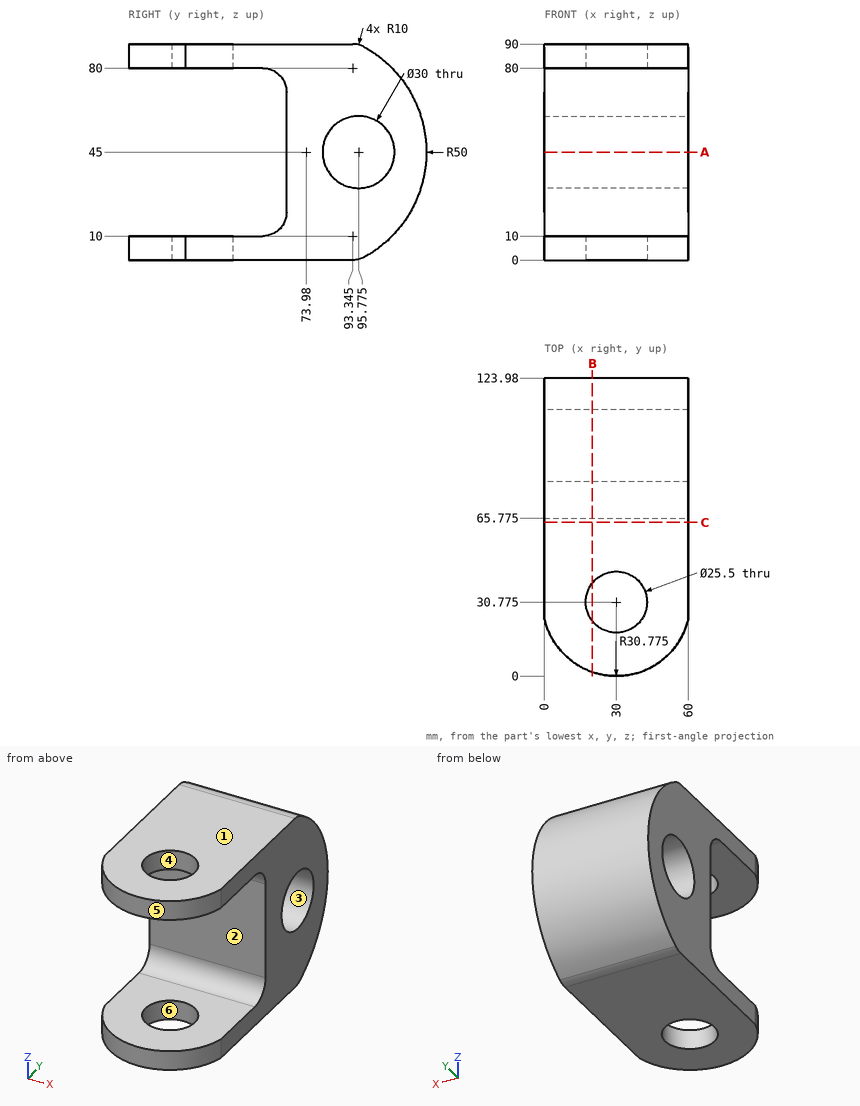
Could you check a few things on this drawing? It's one solid part, dimensions in mm from its lowest x, y, z. A direction names the side the tool comes from. Coordinates: 2 decimals unless noted, no trailing zeros. Loops run counter-clockwise (first coordinate to the right, second up) from the corner with the lowest first, then second, coordinate; pieces in that order, holes last.
1. For the marked faces 1 and 2, which set-ups out of +Z, -Z, +X, -X, +Y, -Y let a thin tool reach every point of the face, with its end or its side?
2. Imagine slicing it at B-B (x = 20). Give the number of separate pieces and of enclosed holes in the cut face, and give its area (3 significant figures).
3. For P1, Ø3, axis at x = 32, z = 9.5, coming from the +Y side; P2, Ø1, axis at x = 14, z = 66, coming from the -Y side (1 decimal); P3, Ø10, axis at x = 11.5, z = 73, coming from the -Y side (1 decimal), each with a flat end and sliding along its axis, tell me the tip position at first contact or that it passes through.
4. Imagine slicing it at C-C (y = 64). Please give me the cut outline in (x, z), and give its area (3 significant figures).
5. Imagine slicing it at A-A (z = 45). Please give me the cut outline in (x, y) (1 decimal).
6. I need wall thicknesses on L1, parallel to Y at x = 33, z = 45 (1 decimal); L2, parallel to Z at x = 46, y = 22.5; L3, parallel to Y at x = 33, z = 83.5 (1 decimal). Which ranges of each line are inside material? Lowest first, please.
7. We'd pull the mould along X, two halves only. Please class the marked faces 3, 4, 5 and 6: released by +X, released by -X, zero draft, split by the parting line, or undercut.
Computed values:
1. face 1: +Z, +X, -X, +Y, -Y
1. face 2: +X, -X, -Y
2. separate pieces: 3
2. enclosed holes: 1
2. area: 4,820 mm2
3. P1: stops at y = 110.64
3. P2: stops at y = 65.8
3. P3: stops at y = 61.8
4. outline: (0, 0) - (60, 0) - (60, 14.31) - (0, 14.31) - close; (0, 75.69) - (60, 75.69) - (60, 90) - (0, 90) - close
4. area: 1,720 mm2
5. outline: (0, 65.8) - (60, 65.8) - (60, 80.8) - (0, 80.8) - close; (0, 110.8) - (60, 110.8) - (60, 124) - (0, 124) - close
6. L1: y = 65.8 to 80.8, 110.8 to 124
6. L2: z = 0 to 10, 80 to 90
6. L3: y = 0.1 to 18.4, 43.2 to 105.9
7. face 3: zero draft
7. face 4: undercut
7. face 5: split by the parting line
7. face 6: undercut
